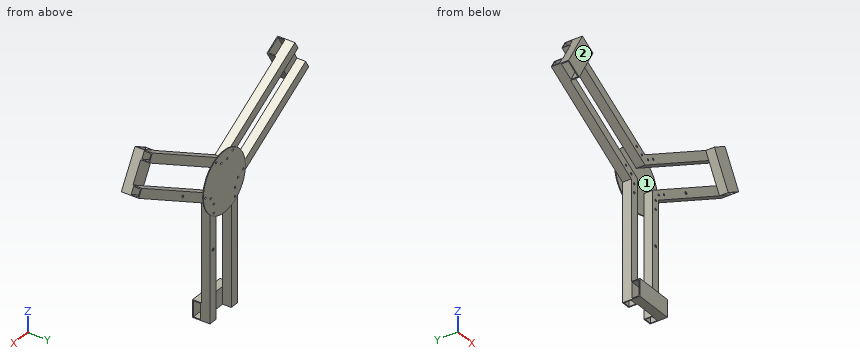
from build123d import *

# Parameters (mm, degrees)
SKETCH6_W             = 25.4
SKETCH6_H             = 25.4
SKETCH6_W_2           = 20.32
SKETCH6_H_2           = 20.32
BOSS_EXTRUDE3_DEPTH   = 363.22
BOSS_EXTRUDE3_2_DEPTH = 363.22
SKETCH7_W             = 50.8
SKETCH7_H             = 25.359897542
SKETCH7_W_2           = 45.72
SKETCH7_H_2           = 20.279897542
BOSS_EXTRUDE4_DEPTH   = 114.3
CUT_EXTRUDE1_DEPTH    = 384.612481677
CUT_EXTRUDE2_DEPTH    = 384.612481677
CIRPATTERN1_COUNT     = 3
SKETCH12_R            = 3
CUT_EXTRUDE3_DEPTH    = 519.942549655
SKETCH13_R            = 87.5
BOSS_EXTRUDE6_DEPTH   = 2
SKETCH14_R            = 3
CUT_EXTRUDE4_DEPTH    = 518.180396616
SKETCH15_R            = 4
CUT_EXTRUDE5_DEPTH    = 519.942549655
SKETCH16_R            = 4
CUT_EXTRUDE6_DEPTH    = 519.942549655


with BuildPart() as part:
    # Sketch6 → Boss-Extrude3 (new body)
    with BuildSketch(Plane.XY.offset(-12.7)):
        with Locations((-44.45, 0)):
            Rectangle(SKETCH6_W, SKETCH6_H)
        with Locations((-44.45, 0)):
            Rectangle(SKETCH6_W_2, SKETCH6_H_2, mode=Mode.SUBTRACT)
    extrude(amount=-BOSS_EXTRUDE3_DEPTH)



with BuildPart() as body_2:
    # Sketch6 → Boss-Extrude3 2 (new body)
    with BuildSketch(Plane.XY.offset(-12.7)):
        with Locations((44.45, 0)):
            Rectangle(SKETCH6_W, SKETCH6_H)
        with Locations((44.45, 0)):
            Rectangle(SKETCH6_W_2, SKETCH6_H_2, mode=Mode.SUBTRACT)
    extrude(amount=-BOSS_EXTRUDE3_2_DEPTH)


with BuildPart() as part_1:
    add(part.part)

    add(body_2.part)  # Boss-Extrude4 merges body 2
    # Sketch7 → Boss-Extrude4 (add)
    with BuildSketch(Plane(origin=(-57.15, 0, 0), x_dir=(0, 0, -1), z_dir=(1, 0, 0))):
        with Locations((350.52, -25.379948771)):
            Rectangle(SKETCH7_W, SKETCH7_H)
        with Locations((350.52, -25.379948771)):
            Rectangle(SKETCH7_W_2, SKETCH7_H_2, mode=Mode.SUBTRACT)
    extrude(amount=BOSS_EXTRUDE4_DEPTH)

    # Sketch9 → Cut-Extrude1 (cut, through all)
    with BuildSketch(Plane(origin=(0, 12.7, 0), x_dir=(1, 0, 0), z_dir=(0, 1, 0))):
        Polygon((0, 0), (66.166370432, 38.20117178), (56.531711502, -13.195312554), align=None)
    extrude(amount=-CUT_EXTRUDE1_DEPTH, mode=Mode.SUBTRACT)

    # Sketch10 → Cut-Extrude2 (cut, through all)
    with BuildSketch(Plane(origin=(0, 12.7, 0), x_dir=(1, 0, 0), z_dir=(0, 1, 0))):
        Polygon((0, 0), (-91.357136084, 52.74506711), (-72.051101597, -19.306034487), align=None)
    extrude(amount=-CUT_EXTRUDE2_DEPTH, mode=Mode.SUBTRACT)


with BuildPart() as cirpattern1_1:
    # CirPattern1: pattern copy
    add(part_1.part.rotate(Axis((0, 0, 0), (0, 1, 0)), 1 * 360 / CIRPATTERN1_COUNT))


with BuildPart() as cirpattern1_2:
    # CirPattern1: pattern copy
    add(part_1.part.rotate(Axis((0, 0, 0), (0, 1, 0)), 2 * 360 / CIRPATTERN1_COUNT))


with BuildPart() as cut_extrude3_tool:
    # Sketch12 → Cut-Extrude3 (new, through all)
    with BuildSketch(Plane(origin=(0, 12.7, 0), x_dir=(1, 0, 0), z_dir=(0, 1, 0))):
        with Locations(Location((44.45, 40.327916303, 0), (0, 0, 90))):
            Circle(SKETCH12_R)
        with Locations(Location((57.15, 18.330871047, 0), (0, 0, 90))):
            Circle(SKETCH12_R)
    extrude(amount=-CUT_EXTRUDE3_DEPTH)


with BuildPart() as part_2:
    add(part_1.part)

    # Cut-Extrude3: cut by cut_extrude3_tool
    add(cut_extrude3_tool.part, mode=Mode.SUBTRACT)


    add(cirpattern1_1.part)  # Boss-Extrude6 merges CirPattern1_1


with BuildPart() as cirpattern1_2_1:
    add(cirpattern1_2.part)

    # Cut-Extrude3: cut by cut_extrude3_tool
    add(cut_extrude3_tool.part, mode=Mode.SUBTRACT)


with BuildPart() as part_3:
    add(part_2.part)

    add(cirpattern1_2_1.part)  # Boss-Extrude6 merges CirPattern1_2
    # Sketch13 → Boss-Extrude6 (add)
    with BuildSketch(Plane(origin=(0, 12.7, 0), x_dir=(1, 0, 0), z_dir=(0, 1, 0))):
        with Locations(Location((0, 0, 0), (0, 0, 68.724233024))):
            Circle(SKETCH13_R)
    extrude(amount=BOSS_EXTRUDE6_DEPTH)

    # Sketch14 → Cut-Extrude4 (cut, through all)
    with BuildSketch(Plane.XZ.offset(12.7)):
        with Locations(Location((57.15, -18.330871047, 0), (0, 0, 270))):
            Circle(SKETCH14_R)
        with Locations(Location((44.45, -40.327916303, 0), (0, 0, 270))):
            Circle(SKETCH14_R)
        with Locations(Location((-57.15, -18.330871047, 0), (0, 0, 270))):
            Circle(SKETCH14_R)
        with Locations(Location((-44.45, -40.327916303, 0), (0, 0, 270))):
            Circle(SKETCH14_R)
        with Locations(Location((12.7, 58.65878735, 0), (0, 0, 270))):
            Circle(SKETCH14_R)
        with Locations(Location((-12.7, 58.65878735, 0), (0, 0, 270))):
            Circle(SKETCH14_R)
        with Locations(Location((44.45, -65.727916303, 0), (0, 0, 270))):
            Circle(SKETCH14_R)
        with Locations(Location((79.147045256, -5.630871047, 0), (0, 0, 270))):
            Circle(SKETCH14_R)
        with Locations(Location((34.697045256, 71.35878735, 0), (0, 0, 270))):
            Circle(SKETCH14_R)
        with Locations(Location((-34.697045256, 71.35878735, 0), (0, 0, 270))):
            Circle(SKETCH14_R)
        with Locations(Location((-79.147045256, -5.630871047, 0), (0, 0, 270))):
            Circle(SKETCH14_R)
        with Locations(Location((-44.45, -65.727916303, 0), (0, 0, 270))):
            Circle(SKETCH14_R)
    extrude(amount=-CUT_EXTRUDE4_DEPTH, mode=Mode.SUBTRACT)

    # Sketch15 → Cut-Extrude5 (cut, through all)
    with BuildSketch(Plane(origin=(0, 12.7, 0), x_dir=(1, 0, 0), z_dir=(0, 1, 0))):
        with Locations(Location((44.45, 170.92, 0), (0, 0, 90))):
            Circle(SKETCH15_R)
    extrude(amount=-CUT_EXTRUDE5_DEPTH, mode=Mode.SUBTRACT)

    # Sketch16 → Cut-Extrude6 (cut, through all)
    with BuildSketch(Plane(origin=(0, 12.7, 0), x_dir=(1, 0, 0), z_dir=(0, 1, 0))):
        with Locations(Location((170.246062015, -46.965170802, 0), (0, 0, 270))):
            Circle(SKETCH16_R)
    extrude(amount=-CUT_EXTRUDE6_DEPTH, mode=Mode.SUBTRACT)


solid = part_3.part
Input: part model. Units: mm. Frame: model coordinates. Face numbers are marked on the shaded views. Coordinates: 2 decimals unless noted, no trailing zeros. Order: outer loops, then holes, each group sorted by start corner. A loop starts at its lowest first (then second) coordinate and runs counter-clockwise, first axis right, second up. Notation, with made-up numbers: M 1.25,79 L 18.25,79 A17 ccw 18.25,107 Z; hole C 60,38.5 d2. An arc over 180 degrees is marked long. Write item = value, one per line. Start each with the question number.
(1) Line query: line 1 along X through (y, z) = (-12.05, -170.92); line 2 along X through (y, z) = (0.5, -262.5); line 3 along Z through (x, y) = (-147.5, -5). Output: solid intervals per line, ascending. Write a range as [from, to].
(2) Section C-C on z = 199.5. Give the number of separate pieces and of enclosed holes in the cut face, and give its area (3 significant figures).
(3) Section B-B on x = -168. Output: boundary loops of the cut face in (y, z), and give its area (3 significant figures).
(4) Section A-A on z = -109. Output: boundary loops of the cut face in (x, y), and give its area (3 significant figures).
(5) Pull-direction query (X, two-part tool) for the marked faces 1 and 2; classes: released by +X, released by -X, zero draft, split by the parting line, or undercut.
(6) First-contact query: P1, Ø1.5, axis at x = 22, z = -39, coming from the -Y side; P2, Ø8, axis at x = -44, y = -24, coming from the +Z side; P3, Ø3, axis at y = 1, z = 79, coming from the -X side. Flat tips, straight axial feed; report the tip coordinate or a pass-through.
Result set:
q1.line_1 = [-57.15, -31.75], [31.75, 40.45], [48.45, 57.15]
q1.line_2 = [-57.15, -54.61], [-34.29, -31.75], [31.75, 34.29], [54.61, 57.15]
q1.line_3 = [19.17, 22.1], [45.56, 48.5], [121.82, 124.75], [148.22, 151.15]
q2.separate_pieces = 2
q2.enclosed_holes = 4
q2.area = 1,760 mm²
q3.outline = M -12.7,31 L 12.7,31 L 12.7,60.33 L -12.7,60.33 Z; M -12.7,133.66 L 12.7,133.66 L 12.7,162.99 L -12.7,162.99 Z; hole M -10.16,33.94 L 10.16,33.94 L 10.16,57.4 L -10.16,57.4 Z; hole M -10.16,136.59 L 10.16,136.59 L 10.16,160.05 L -10.16,160.05 Z
q3.area = 536 mm²
q4.outline = M -57.15,-12.7 L -31.75,-12.7 L -31.75,12.7 L -57.15,12.7 Z; M 31.75,-12.7 L 57.15,-12.7 L 57.15,12.7 L 31.75,12.7 Z; hole M -54.61,-10.16 L -34.29,-10.16 L -34.29,10.16 L -54.61,10.16 Z; hole M 34.29,-10.16 L 54.61,-10.16 L 54.61,10.16 L 34.29,10.16 Z
q4.area = 465 mm²
q5.face_1 = undercut
q5.face_2 = zero draft
q6.P1 = 12.7
q6.P2 = -325.12
q6.P3 = -253.73
